from build123d import *

# Parameters (mm, degrees)
F1_DEPTH      = 20
F1_DEPTH_BACK = 20
F2_R          = 1.5
F3_DEPTH      = 10
F5_DEPTH      = 3
F6_R          = 1
F7_R          = 1


with BuildPart() as f1:
    # F0 (on Right) → F1 (new body, two sides)
    with BuildSketch(Plane.YZ) as f1_sk:
        with BuildLine():
            Line((-5, 0), (0, 0))
            Line((0, 0), (5, 0))
            Line((5, 0), (4.0900496281, 9.099503719))
            ThreePointArc((4.0900496281, 9.099503719), (3.7660177586, 9.7414525336), (3.0950124379, 10))
            Line((3.0950124379, 10), (0, 10))
            Line((0, 10), (-3.0950124379, 10))
            ThreePointArc((-3.0950124379, 10), (-3.7660177586, 9.7414525336), (-4.0900496281, 9.099503719))
            Line((-4.0900496281, 9.099503719), (-5, 0))
        make_face()
    extrude(amount=F1_DEPTH)
    extrude(f1_sk.sketch, amount=-F1_DEPTH_BACK)

    # F2 (on face) → F3 (cut, through all)
    with BuildSketch(Plane.XY.offset(10)):
        with Locations((-15, 0)):
            Circle(F2_R)
        with Locations((15, 0)):
            Circle(F2_R)
        Circle(F2_R)
    extrude(amount=-F3_DEPTH, mode=Mode.SUBTRACT)

    # F4 (on face) → F5 (cut)
    with BuildSketch(Plane.XY.offset(10)):
        Polygon((-12.3749576506, 1.4532932788), (-14.9460677239, 3), (-17.5711100733, 1.5467067212), (-17.6250423494, -1.4532932788), (-15.0539322761, -3), (-12.4288899267, -1.5467067212), align=None)
        Polygon((17.5711100733, 1.5467067212), (14.9460677239, 3), (12.3749576506, 1.4532932788), (12.4288899267, -1.5467067212), (15.0539322761, -3), (17.6250423494, -1.4532932788), align=None)
        Polygon((1.5, 2.5980762114), (-1.5, 2.5980762114), (-3, 0), (-1.5, -2.5980762114), (1.5, -2.5980762114), (3, 0), align=None)
    extrude(amount=-F5_DEPTH, mode=Mode.SUBTRACT)

    # F6
    f6_edges = [f1.edges().sort_by_distance(p)[0] for p in [
        (20, 0, 10),
    ]]
    fillet(f6_edges, radius=F6_R)

    # F7
    f7_edges = [f1.edges().sort_by_distance(p)[0] for p in [
        (-20, 0, 10),
    ]]
    fillet(f7_edges, radius=F7_R)


solid = f1.part
Geometry check sheet. Reference: the model listing, model coordinates, mm. A direction names the side the tool comes from. Give positions to 0.01 mm unless a question says otherwise; leave off trailing zeros. Loops run counter-clockwise (first coordinate to the right, second up) from the corner with the lowest first, then second, coordinate; pieces in that order, holes last. Notation, with made-up numbers: M 66,-32 L 108,-32 A17 ccw 108,-2 Z; hole C -37.75,38 d6. An arc over 180 degrees is marked long. Answer as a JSON object with one key per item and string values. Group by question number.
Item 1: Gauge pin test, flat ends, axial feed: pin 1 (1.6 mm diameter, centred on x = -16, y = 0.5, fed in from +Z); pin 2 (1.5 mm diameter, centred on x = 0.5, z = 9, fed in from -Y) (3 decimals); pin 3 (2 mm diameter, centred on x = -7.5, z = 2, fed in from -Y); pin 4 (4 mm diameter, centred on x = 14, y = -0.5, fed in from +Z). Record the tip position at first contact, or that the pin passes through.
Item 2: Sectioned sample at C-C on z = 9.5. Record the boundary of the cut face in (x, y).
Item 3: Material ranges on L1, parallel to X at y = -1.25, z = 8; L2, parallel to X at y = -2.5, z = 9.25; L3, parallel to Y at x = -15, z = 2, recorded low to high.
Item 4: Access from +Z, -Z, +X, -X, +Y, -Y to the whole of each face (thin tool, end or side, straight path). Record for faces 1 (the cylindrical face through (-19.715, 4.239, 4.584)), 2 (the flat face through (16.28, 2.26, 8.52)).
Item 5: Mould release check, pull along Y, two halves, no side actions. Record for faces 3 (the flat face through (13.72, -2.26, 8.52)), 4 (the cylindrical face through (0.266, 3.774, 9.735)), 5 (the flat face through (0, 2, 0)): pulls with the +Y half, pulls with the -Y half, needs draft (parallel to the pull), parting line crosses it, or undercut.
Item 6: Sectioned sample at A-A on x = 0. Record the boundary of the cut face in (y, z), plus the area to 3 significant figures.
Item 7: Sectioned sample at B-B on x = 12. Record the boundary of the cut face in (y, z).
Item 8: Sectioned sample at D-D on z = 4.5. Give the number of separate pieces and of enclosed holes in the cut face, plus the area to 3 significant figures.
Findings below:
{
 "1": {"pin 1": "z = 7", "pin 2": "y = -4.175", "pin 3": "y = -4.9", "pin 4": "z = 10"},
 "2": {"outline": "M -19.87,-3.1 A0.87 ccw -19,-3.96 L 19,-3.96 A0.87 ccw 19.87,-3.1 L 19.87,3.1 A0.87 ccw 19,3.96 L -19,3.96 A0.87 ccw -19.87,3.1 Z; hole M -17.63,-1.45 L -15.05,-3 L -12.43,-1.55 L -12.37,1.45 L -14.95,3 L -17.57,1.55 Z; hole M -3,0 L -1.5,-2.6 L 1.5,-2.6 L 3,0 L 1.5,2.6 L -1.5,2.6 Z; hole M 12.37,1.45 L 12.43,-1.55 L 15.05,-3 L 17.63,-1.45 L 17.57,1.55 L 14.95,3 Z"},
 "3": {"L1": "-20 to -17.62, -12.42 to -2.28, 2.28 to 12.42, 17.62 to 20", "L2": "-19.97 to -15.89, -14.15 to -1.56, 1.56 to 14.15, 15.89 to 19.97", "L3": "-4.8 to -1.5, 1.5 to 4.8"},
 "4": {"face 1": "+Z, -X, +Y", "face 2": "+Z"},
 "5": {"face 3": "undercut", "face 4": "pulls with the +Y half", "face 5": "needs draft"},
 "6": {"outline": "M -5,0 L -1.5,0 L -1.5,7 L -2.6,7 L -2.6,10 L -3.1,10 A1 ccw -4.09,9.1 Z; M 1.5,0 L 5,0 L 4.09,9.1 A1 ccw 3.1,10 L 2.6,10 L 2.6,7 L 1.5,7 Z", "area": "53.1 mm2"},
 "7": {"outline": "M -5,0 L 5,0 L 4.09,9.1 A1 ccw 3.1,10 L -3.1,10 A1 ccw -4.09,9.1 Z"},
 "8": {"separate pieces": "1", "enclosed holes": "3", "area": "342 mm2"}
}
